Source: three-view drawing plus pictorial views. Frame: mm from the lowest corner of the part. A direction names the side the tool comes from. Give positions to 0.01 mm unless a question says otherwise; leave off trailing zeros. Loops run counter-clockwise (first coordinate to the right, second up) from the corner with the lowest first, then second, coordinate; pieces in that order, holes last. Notation, with made-up numbers: M 5.5,-13 L 31.5,-13 A16 ccw 31.5,-3 Z; hole C 57,86 d11. An arc over 180 degrees is marked long. Answer as a JSON object with one key per item and string values. Group by question number.
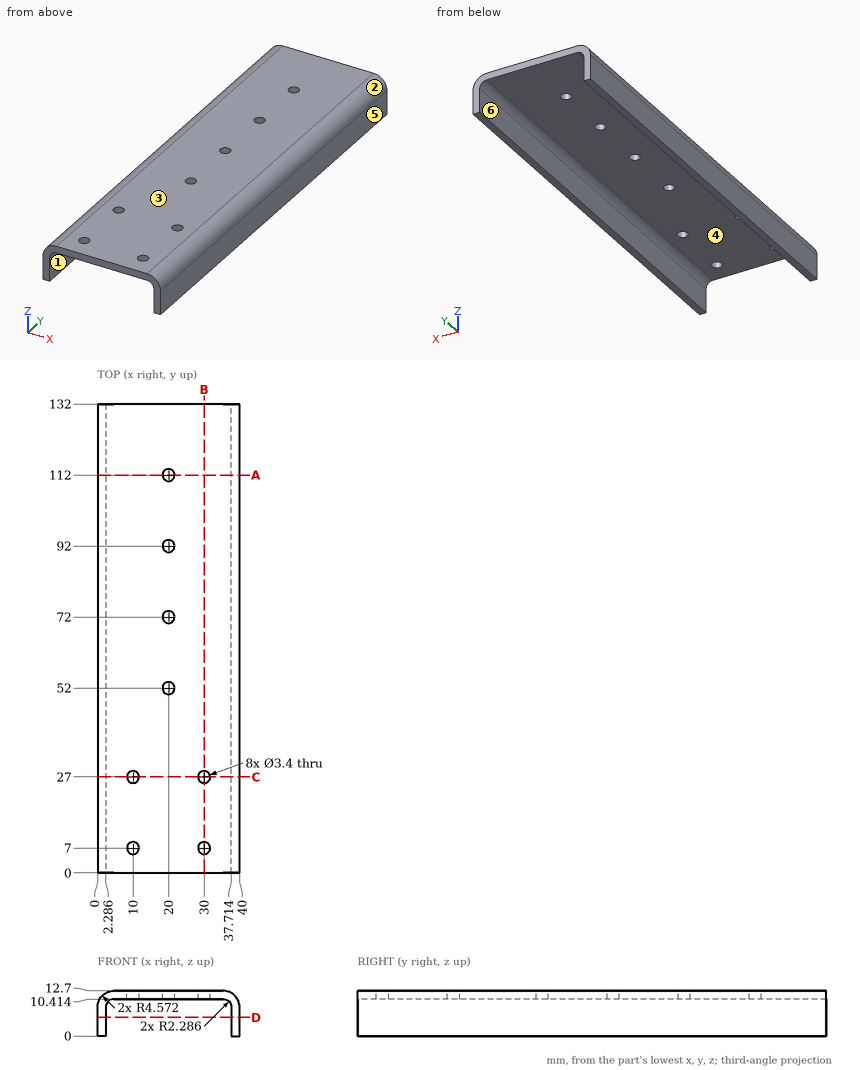
1. Section A-A (y = 112). Output: boundary loops of the cut face in (x, z).
2. Section C-C (y = 27). Output: boundary loops of the cut face in (x, z), then the cut area to 3 significant figures.
3. Section D-D (z = 5.25). Output: boundary loops of the cut face in (x, y), then the cut area to 3 significant figures.
4. Material intervals for L1, parallel to Y at x = 10, z = 11.2; L2, parallel to Y at x = 20, z = 11.2; L3, parallel to X at y = 80, z = 1.75, sorted ascending.
5. First-contact query: P1, Ø8, axis at x = 17.5, y = 38.5, coming from the -Z side; P2, Ø1.5, axis at x = 10, z = 9.5, coming from the +Y side; P3, Ø2, axis at y = 34.5, z = 9, coming from the +X side; P4, Ø1.5, axis at y = 65.5, z = 10, coming from the -X side. Flat tips, straight axial feed; report the tip coordinate or a pass-through.
6. Reachability of the marked faces 1 and 2 from +Z, -Z, +X, -X, +Y, -Y: full face, straight path, thin tool, end or side. Return the list, or none.
7. Mould query, pull axis X, two halves, no side actions, for the marked faces 3, 4, 5 and 6. Classes: pulls with the +X half, pulls with the -X half, needs draft (parallel to the pull), parting line crosses it, or undercut.
8. Section B-B (x = 30). Output: boundary loops of the cut face in (y, z), then the cut area to 3 significant figures.
Geometry results:
{
 "1": {"outline": "M 0,0 L 2.29,0 L 2.29,8.13 A2.29 cw 4.57,10.41 L 18.3,10.41 L 18.3,12.7 L 4.57,12.7 A4.57 ccw 0,8.13 Z; M 21.7,10.41 L 35.43,10.41 A2.29 cw 37.71,8.13 L 37.71,0 L 40,0 L 40,8.13 A4.57 ccw 35.43,12.7 L 21.7,12.7 Z"},
 "2": {"outline": "M 0,0 L 2.29,0 L 2.29,8.13 A2.29 cw 4.57,10.41 L 8.3,10.41 L 8.3,12.7 L 4.57,12.7 A4.57 ccw 0,8.13 Z; M 11.7,10.41 L 28.3,10.41 L 28.3,12.7 L 11.7,12.7 Z; M 31.7,10.41 L 35.43,10.41 A2.29 cw 37.71,8.13 L 37.71,0 L 40,0 L 40,8.13 A4.57 ccw 35.43,12.7 L 31.7,12.7 Z", "area": "117 mm2"},
 "3": {"outline": "M 0,0 L 2.29,0 L 2.29,132 L 0,132 Z; M 37.71,0 L 40,0 L 40,132 L 37.71,132 Z", "area": "604 mm2"},
 "4": {"L1": "0 to 5.3, 8.7 to 25.3, 28.7 to 132", "L2": "0 to 50.3, 53.7 to 70.3, 73.7 to 90.3, 93.7 to 110.3, 113.7 to 132", "L3": "0 to 2.29, 37.71 to 40"},
 "5": {"P1": "z = 10.41", "P2": "through", "P3": "x = 40", "P4": "x = 0.14"},
 "6": {"face 1": "-Z, +Y, -Y", "face 2": "+Z, +X, +Y, -Y"},
 "7": {"face 3": "needs draft", "face 4": "undercut", "face 5": "pulls with the +X half", "face 6": "undercut"},
 "8": {"outline": "M 0,10.41 L 5.3,10.41 L 5.3,12.7 L 0,12.7 Z; M 8.7,10.41 L 25.3,10.41 L 25.3,12.7 L 8.7,12.7 Z; M 28.7,10.41 L 132,10.41 L 132,12.7 L 28.7,12.7 Z", "area": "286 mm2"}
}
